```python
from build123d import *

# Parameters (mm, degrees)
F0_W     = 80
F0_H     = 50
F1_DEPTH = 40
F2_R     = 7
F3_DEPTH = 15
F4_T     = -2.5
F5_R     = 5


with BuildPart() as f1:
    # F0 (on Top) → F1 (new body)
    with BuildSketch(Plane.XY):
        Rectangle(F0_W, F0_H)
    extrude(amount=F1_DEPTH)

    # F2 (on face) → F3 (join)
    with BuildSketch(Plane.XY.offset(40)):
        Circle(F2_R)
    extrude(amount=F3_DEPTH)

    # F4
    f4_openings = [f1.faces().sort_by_distance(p)[0] for p in [
        (0, 0, 55),
    ]]
    offset(amount=F4_T, openings=f4_openings, kind=Kind.INTERSECTION)

    # F5
    f5_edges = [f1.edges().sort_by_distance(p)[0] for p in [
        (-7, 0, 40),
        (0, -25, 40),
        (40, 0, 40),
        (-40, 0, 40),
        (0, 25, 40),
        (-40, -25, 20),
        (40, -25, 20),
        (-40, 25, 20),
        (40, 25, 20),
    ]]
    fillet(f5_edges, radius=F5_R)


solid = f1.part
```
For this review, take the finished solid that the model builds, in its own axes (mm). A direction names the side the tool comes from. Round coordinates to 2 decimals unless told otherwise and drop trailing zeros. Write each loop counter-clockwise with the first axis right and the second up, starting at its lowest first coordinate (ties: lowest second). Pieces come first, ordered by that corner, then holes. Notation, with made-up numbers: (-35, -19) -> (19, -19) arc R21 ccw to (19, 18) -> close; hole circle Ø3 at (87.5, -23.5). An arc over 180 degrees is marked (long way). Use one line per item in the form item = value.
1) Take a section at A-A, the plane y = -14. Write out the cut boundary in (x, z).
Found:
outline = (-40, 0) -> (40, 0) -> (40, 35) arc R5 ccw to (35, 40) -> (-35, 40) arc R5 ccw to (-40, 35) -> close; hole (-37.5, 2.5) -> (37.5, 2.5) -> (37.5, 37.5) -> (-37.5, 37.5) -> close
2) To check wall thickness, follow L1, parallel to Z at x = -17, y = -2; L2, parallel to Y at x = 0, z = 46.5; L3, parallel to X at y = -13.5, z = 9. State the ranges of each line that lie inside material, in increasing order. Write a range as from..to.
Found:
L1 = 0..2.5, 37.5..40
L2 = -7..-4.5, 4.5..7
L3 = -40..-37.5, 37.5..40
3) Take a section at B-B, the plane z = 8. Write out the cut boundary in (x, y).
Found:
outline = (-40, -20) arc R5 ccw to (-35, -25) -> (35, -25) arc R5 ccw to (40, -20) -> (40, 20) arc R5 ccw to (35, 25) -> (-35, 25) arc R5 ccw to (-40, 20) -> close; hole (-37.5, -22.5) -> (37.5, -22.5) -> (37.5, 22.5) -> (-37.5, 22.5) -> close
4) Take a section at C-C, the plane y = 0. Write out the cut boundary in (x, z).
Found:
outline = (-40, 0) -> (40, 0) -> (40, 35) arc R5 ccw to (35, 40) -> (12, 40) arc R5 cw to (7, 45) -> (7, 55) -> (4.5, 55) -> (4.5, 37.5) -> (37.5, 37.5) -> (37.5, 2.5) -> (-37.5, 2.5) -> (-37.5, 37.5) -> (-4.5, 37.5) -> (-4.5, 55) -> (-7, 55) -> (-7, 45) arc R5 cw to (-12, 40) -> (-35, 40) arc R5 ccw to (-40, 35) -> close
5) Tool access review of faces 1 (the cylindrical face through (-39, 23, 18)), 2 (the flat face through (-1, 0, 2.5)), 3 (the cylindrical face through (6.466, -2.681, 49.93)): name each direction out of +Z, -Z, +X, -X, +Y, -Y from which nothing blocks a thin tool from reaching the whole face with its end or side.
Found:
face_1 = +Z, -Z, -X, +Y
face_2 = none
face_3 = +Z
6) Take a section at D-D, the plane x = -17. Write out the cut boundary in (y, z).
Found:
outline = (-25, 0) -> (25, 0) -> (25, 35) arc R5 ccw to (20, 40) -> (-20, 40) arc R5 ccw to (-25, 35) -> close; hole (-22.5, 2.5) -> (22.5, 2.5) -> (22.5, 37.5) -> (-22.5, 37.5) -> close
7) Mouldability with a two-part tool opening along Z and no side actions: class faces 4 (the cylindrical face through (0, 24, 38)), 5 (the cylindrical face through (-0.59, 4.46, 46.13)), 6 (the flat face through (-37.5, 0, 20)) as +Z half, -Z half, draft (parallel to the pull), parting line (faces both ways), or undercut.
Found:
face_4 = +Z half
face_5 = draft
face_6 = undercut
